Can you work these out from the model? Positions are in its coordinate system, mm. Face numbers are marked on the shaded views. A direction names the side the tool comes from. Coordinates: 2 decimals unless noted, no trailing zeros. Order: outer loops, then holes, each group sorted by start corner. A loop starts at its lowest first (then second) coordinate and runs counter-clockwise, first axis right, second up. Notation, with made-up numbers: (-1.5, -17) -> (14.5, -17) arc R27 ccw to (14.5, 16) -> close; hole circle Ø4 at (70, 65). An arc over 180 degrees is marked (long way). Answer in a Markdown table with one row per item.
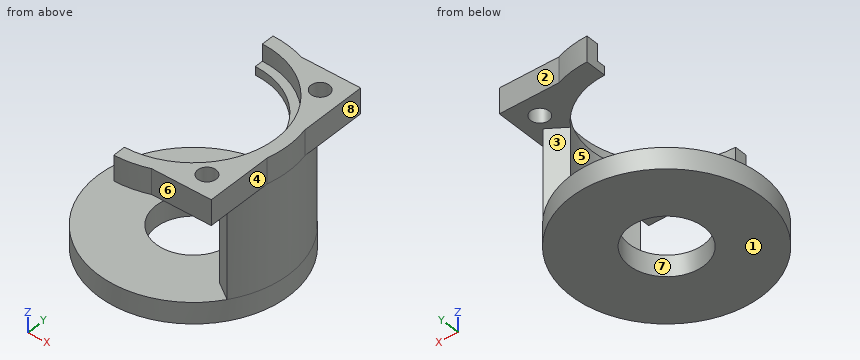
```python
from build123d import *

# Parameters (mm, degrees)
SKETCH1_R           = 22.4995417
SKETCH1_R_2         = 17.4995417
BOSS_EXTRUDE1_DEPTH = 6
CUT_EXTRUDE1_START  = -4
SKETCH2_R           = 19.4995417
SKETCH2_R_2         = 17.4995417
CUT_EXTRUDE1_DEPTH  = 4
BOSS_EXTRUDE2_DEPTH = 6
BOSS_EXTRUDE3_START = 24
BOSS_EXTRUDE3_DEPTH = 24
BOSS_EXTRUDE4_START = 5
SKETCH6_R           = 22.4995417
SKETCH6_R_2         = 8.79453705
BOSS_EXTRUDE4_DEPTH = 5
CUT_EXTRUDE2_DEPTH  = 44.051814752
SKETCH9_R           = 2.165
CUT_EXTRUDE4_DEPTH  = 44.051814752


with BuildPart() as part:
    # Sketch1 → Boss-Extrude1 (new body)
    with BuildSketch(Plane.XY):
        Circle(SKETCH1_R)
        Circle(SKETCH1_R_2, mode=Mode.SUBTRACT)
    extrude(amount=BOSS_EXTRUDE1_DEPTH)

    # Sketch2 → Cut-Extrude1 (cut)
    with BuildSketch(Plane.XY.offset(6).offset(CUT_EXTRUDE1_START)):
        Circle(SKETCH2_R)
        Circle(SKETCH2_R_2, mode=Mode.SUBTRACT)
    extrude(amount=CUT_EXTRUDE1_DEPTH, mode=Mode.SUBTRACT)

    # Sketch3 → Boss-Extrude2 (add, through all)
    with BuildSketch(Plane(origin=(0, 0, 0), x_dir=(-1, 0, 0), z_dir=(0, 0, -1))):
        with BuildLine():
            Line((-7.783576547, 21.11031295), (-21.864631522, 21.11031295))
            Line((-21.864631522, 21.11031295), (-21.864631522, 5.307284156))
            ThreePointArc((-21.864631522, 5.307284156), (-16.798452018, 14.96801211), (-7.783576547, 21.11031295))
        make_face()
        with BuildLine():
            Line((21.864631522, -21.11031295), (7.783576547, -21.11031295))
            ThreePointArc((7.783576547, -21.11031295), (16.798452018, -14.96801211), (21.864631522, -5.307284156))
            Line((21.864631522, -5.307284156), (21.864631522, -21.11031295))
        make_face()
        with BuildLine():
            Line((21.864631522, 21.11031295), (7.783576547, 21.11031295))
            ThreePointArc((7.783576547, 21.11031295), (16.798452018, 14.96801211), (21.864631522, 5.307284156))
            Line((21.864631522, 5.307284156), (21.864631522, 21.11031295))
        make_face()
        with BuildLine():
            Line((-21.864631522, -21.11031295), (-21.864631522, -5.307284156))
            ThreePointArc((-21.864631522, -5.307284156), (-16.798452018, -14.96801211), (-7.783576547, -21.11031295))
            Line((-7.783576547, -21.11031295), (-21.864631522, -21.11031295))
        make_face()
    extrude(amount=-BOSS_EXTRUDE2_DEPTH)

    # Sketch5 → Boss-Extrude3 (add)
    with BuildSketch(Plane(origin=(0, 0, 0), x_dir=(-1, 0, 0), z_dir=(0, 0, -1)).offset(BOSS_EXTRUDE3_START)):
        with BuildLine():
            Line((-14.441527519, 9.883129191), (-18.5677863, 12.706954341))
            ThreePointArc((-18.5677863, 12.706954341), (-22.4995417, 0), (-18.5677863, -12.706954341))
            Line((-18.5677863, -12.706954341), (-14.441527519, -9.883129191))
            ThreePointArc((-14.441527519, -9.883129191), (-17.4995417, 0), (-14.441527519, 9.883129191))
        make_face()
    extrude(amount=-BOSS_EXTRUDE3_DEPTH)

    # Sketch6 → Boss-Extrude4 (add)
    with BuildSketch(Plane(origin=(0, 0, -24), x_dir=(-1, 0, 0), z_dir=(0, 0, -1)).offset(BOSS_EXTRUDE4_START)):
        Circle(SKETCH6_R)
        Circle(SKETCH6_R_2, mode=Mode.SUBTRACT)
    extrude(amount=-BOSS_EXTRUDE4_DEPTH)

    # Sketch7 → Cut-Extrude2 (cut, through all)
    with BuildSketch(Plane(origin=(0, 0, 0), x_dir=(-1, 0, 0), z_dir=(0, 0, -1))):
        Polygon((0, 20.425006128), (0, -31.813494394), (36.314088068, -29.010206824), (38.071070197, 28.399979516), (-0.660202218, 29.585311907), (0, 25.789149152), align=None)
    extrude(amount=-CUT_EXTRUDE2_DEPTH, mode=Mode.SUBTRACT)

    # Sketch9 → Cut-Extrude4 (cut, through all)
    with BuildSketch(Plane(origin=(0, 0, 0), x_dir=(-1, 0, 0), z_dir=(0, 0, -1))):
        with Locations((16.571715691, 16)):
            Circle(SKETCH9_R)
        with Locations((16.571715691, -16)):
            Circle(SKETCH9_R)
        with Locations((-16.571715691, -16)):
            Circle(SKETCH9_R)
        with Locations((-16.571715691, 16)):
            Circle(SKETCH9_R)
    extrude(amount=-CUT_EXTRUDE4_DEPTH, mode=Mode.SUBTRACT)


solid = part.part
```
(1) I need wall thicknesses on line 1 (Z direction, x = 14, y = -13.5); line 2 (Z direction, x = 1.5, y = 20); line 3 (Y direction, x = 0, z = -25.2). Which ranges of each line are inside material? Lowest first, please. Write a range as [from, to].
Response values:
| item | result |
|---|---|
| line 1 | [-29, -24], [0, 2] |
| line 2 | [-29, -24], [0, 6] |
| line 3 | [-22.5, -8.79], [8.79, 22.5] |
(2) Suppose I cut it at B-B (x = -7.5). Please give me the cut outline in (y, z), and give its area (3 significant figures).
Response values:
| item | result |
|---|---|
| outline | (-21.21, -29) -> (-4.59, -29) -> (-4.59, -24) -> (-21.21, -24) -> close; (4.59, -29) -> (21.21, -29) -> (21.21, -24) -> (4.59, -24) -> close |
| area | 166 mm2 |
(3) We'd pull the mould along Y, two halves only. Please class the marked faces 5, 6, 7 and 8: +Y half, -Y half, draft (parallel to the pull), parting line (faces both ways), or undercut.
Response values:
| item | result |
|---|---|
| face 5 | undercut |
| face 6 | -Y half |
| face 7 | undercut |
| face 8 | draft |
(4) Suppose I cut it at C-C (x = 1.5). Please give me the cut outline in (y, z), and give its area (3 significant figures).
Response values:
| item | result |
|---|---|
| outline | (-22.45, -29) -> (-8.67, -29) -> (-8.67, -24) -> (-22.45, -24) -> close; (-22.45, 0) -> (-17.44, 0) -> (-17.44, 2) -> (-19.44, 2) -> (-19.44, 6) -> (-22.45, 6) -> close; (8.67, -29) -> (22.45, -29) -> (22.45, -24) -> (8.67, -24) -> close; (17.44, 0) -> (22.45, 0) -> (22.45, 6) -> (19.44, 6) -> (19.44, 2) -> (17.44, 2) -> close |
| area | 182 mm2 |
(5) Suppose I cut it at D-D (y = -16). Please give me the cut outline in (x, z), and give its area (3 significant figures).
Response values:
| item | result |
|---|---|
| outline | (-15.82, -29) -> (15.82, -29) -> (15.82, -24) -> (-15.82, -24) -> close; (7.09, 0) -> (14.41, 0) -> (14.41, 6) -> (11.15, 6) -> (11.15, 2) -> (7.09, 2) -> close; (18.74, 0) -> (21.86, 0) -> (21.86, 6) -> (18.74, 6) -> close |
| area | 205 mm2 |
(6) Will these pins go through, and if not, where does the flat tip stop? pin 1 Ø1 at (y, z) = (-8.5, -10.5) entering from -X; pin 2 Ø9.5 at (x, y) = (5.5, 3.5) entering from +Z; pin 3 Ø3 at (y, z) = (8.5, -20) entering from -X.
Response values:
| item | result |
|---|---|
| pin 1 | x = 15.01 |
| pin 2 | z = -24 |
| pin 3 | x = 14.44 |
(7) Suppose I cut it at A-A (y = 0). Please give me the cut outline in (x, z), and give its area (3 significant figures).
Response values:
| item | result |
|---|---|
| outline | (-22.5, -29) -> (-8.79, -29) -> (-8.79, -24) -> (-22.5, -24) -> close; (8.79, -29) -> (22.5, -29) -> (22.5, 6) -> (19.5, 6) -> (19.5, 2) -> (17.5, 2) -> (17.5, -24) -> (8.79, -24) -> close |
| area | 279 mm2 |
(8) On a 3-axis mill with a long thin cutter (end or side, diameter ignored), from which of +Z, -Z, +X, -X, +Y, -Y can I reach the whole of each face in a straight line? I mean the marked faces 1, 2, 3 and 4. Say none if no direction works.
Response values:
| item | result |
|---|---|
| face 1 | -Z, +X, -X, +Y, -Y |
| face 2 | +Z, -Z, +X, +Y |
| face 3 | -X, +Y |
| face 4 | +Z, -Z, +X, -Y |
